Part print with two shaded views. Sizes in mm from the minimum x, y, z corner. A direction names the side the tool comes from. Coordinates: 2 decimals unless noted, no trailing zeros. Loops run counter-clockwise (first coordinate to the right, second up) from the corner with the lowest first, then second, coordinate; pieces in that order, holes last. Notation, with made-up numbers: (40.25, 32.5) -> (93.25, 32.5) arc R12 cw to (93.25, 55.5) -> close; hole circle Ø8 at (10.25, -15). An arc over 180 degrees is marked (long way). Write each question's results on one line, items separated by ' | '.
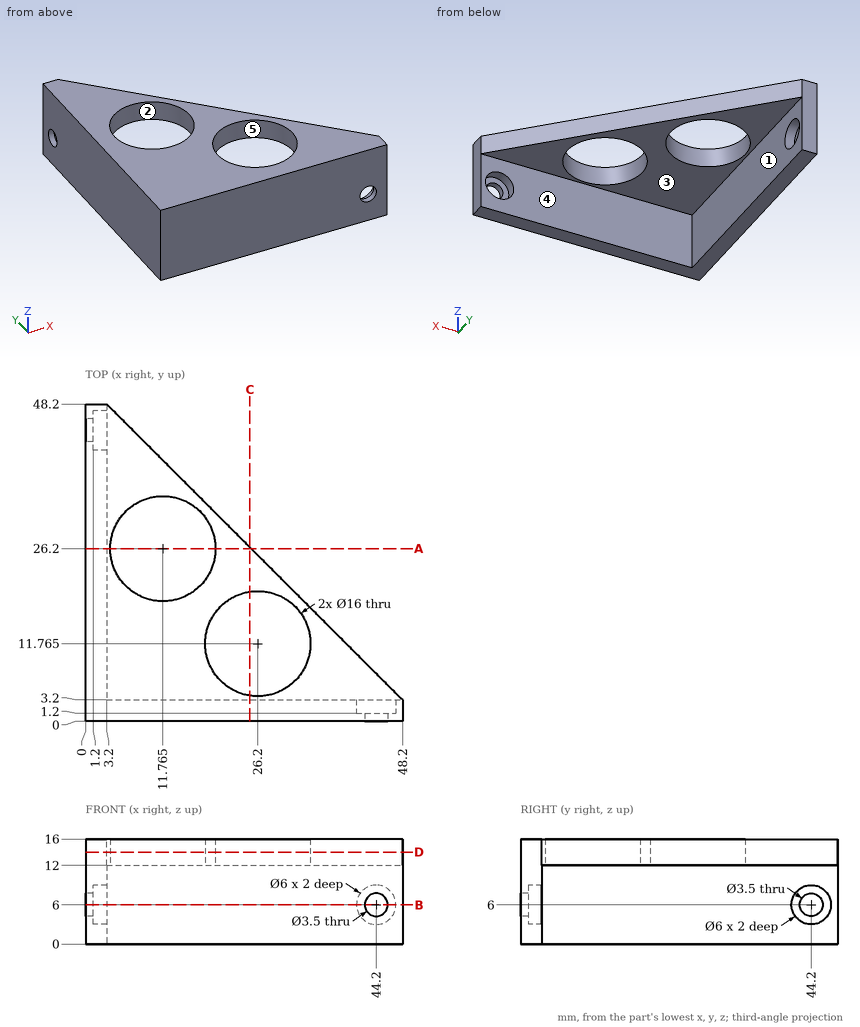
Q1. Cut at A-A on y = 26.2. Write the cut outline in (x, z) (3 decimals).
Results are:
outline: (0, 0) -> (3.2, 0) -> (3.2, 12) -> (3.765, 12) -> (3.765, 16) -> (0, 16) -> close; (19.765, 12) -> (25.2, 12) -> (25.2, 16) -> (19.765, 16) -> close
Q2. Cut at B-B on z = 6. Write the cut outline in (x, y).
Results are:
outline: (0, 0) -> (42.45, 0) -> (42.45, 1.2) -> (41.2, 1.2) -> (41.2, 3.2) -> (3.2, 3.2) -> (3.2, 41.2) -> (1.2, 41.2) -> (1.2, 42.45) -> (0, 42.45) -> close; (0, 45.95) -> (1.2, 45.95) -> (1.2, 47.2) -> (3.2, 47.2) -> (3.2, 48.2) -> (0, 48.2) -> close; (45.95, 0) -> (48.2, 0) -> (48.2, 3.2) -> (47.2, 3.2) -> (47.2, 1.2) -> (45.95, 1.2) -> close
Q3. Cut at D-D on z = 14. Write the cut outline in (x, y) (3 decimals), and give its area (3 significant figures).
Results are:
outline: (0, 0) -> (48.2, 0) -> (48.2, 3.2) -> (3.2, 48.2) -> (0, 48.2) -> close; hole circle Ø16 at (11.765, 26.2); hole circle Ø16 at (26.2, 11.765) | area: 909 mm^2
Q4. Cut at C-C on x = 25. Write the cut outline in (y, z), and give its area (3 significant figures).
Results are:
outline: (0, 0) -> (3.2, 0) -> (3.2, 12) -> (3.86, 12) -> (3.86, 16) -> (0, 16) -> close; (19.67, 12) -> (26.4, 12) -> (26.4, 16) -> (19.67, 16) -> close | area: 80.7 mm^2
Q5. Pull direction Y, two halves, no side cores. Call the marked faces 3, 4 and 5: +Y half, -Y half, draft (parallel to the pull), parting line (faces both ways), or undercut.
Results are:
face 3: draft | face 4: +Y half | face 5: undercut
Q6. Drop flat-ended pins along their axis: pin 1 (3 mm diameter, centred on x = 43, z = 7.5, fed in from +Y); pin 2 (6 mm diameter, centred on y = 35.5, z = 6.5, fed in from +X); pin 3 (14.5 mm diameter, centred on x = 11.765, y = 26.2, fed in from -Z); pin 4 (22.5 mm diameter, centred on x = 28.5, y = 28, fed in from -Z). Give the stop position or say it passes through.
Results are:
pin 1: y = 3.2 | pin 2: x = 3.2 | pin 3: through | pin 4: z = 12
Q7. Which spindle directions (+Z, -Z, +X, -X, +Y, -Y) get a long thin tool onto all of the face, cutting with end or side? Do the marked faces 1 and 2. Say none if no direction does.
Results are:
face 1: -Z, +X, +Y | face 2: +Z, -Z
Q8. Wall check: L1, parallel to Y at x = 0.9, z = 6; L2, parallel to Z at x = 0.85, y = 44.2; L3, parallel to Z at x = 44.2, y = 2.7. Give the ranges that are in metal, low to high. Write a range as from..to.
Results are:
L1: 0..42.45, 45.95..48.2 | L2: 0..4.25, 7.75..16 | L3: 0..3, 9..16
